The listing builds one solid part. Answer for the finished solid, in the listing's coordinates (mm). Coordinates: 2 decimals unless noted, no trailing zeros. Order: outer loops, then holes, each group sorted by start corner. A loop starts at its lowest first (then second) coordinate and runs counter-clockwise, first axis right, second up.
from build123d import *

# Parameters (mm, degrees)
F0_W     = 8
F0_H     = 8
F0_W_2   = 7.999141
F1_DEPTH = 3
F2_R     = 2.2
F3_DEPTH = 5
F4_R     = 2.5
F5_DEPTH = 6.5


with BuildPart() as f1:
    # F0 (on Top) → F1 (new body)
    with BuildSketch(Plane.XY):
        Polygon((-37.766442, 20.223286), (-40, 20.223286), (-40, -20.223286), (-37.766442, -20.223286), (-29.767301, -20.223286), (29.767301, -20.223286), (37.766442, -20.223286), (40, -20.223286), (40, 20.223286), (37.766442, 20.223286), (36.185599, 20.223286), (29.766442, 20.223286), (28.185599, 20.223286), (-29.766442, 20.223286), align=None)
        with Locations((-33.766442, 24.223286)):
            Rectangle(F0_W, F0_H)
        with Locations((-33.766872, -24.223286)):
            Rectangle(F0_W_2, F0_H)
        Polygon((29.766442, 28.223286), (29.766442, 20.223286), (36.185599, 20.223286), (37.766442, 20.223286), (37.766442, 28.223286), align=None)
        with Locations((33.766872, -24.223286)):
            Rectangle(F0_W_2, F0_H)
    extrude(amount=F1_DEPTH)

    # F2 (on Top) → F3 (cut)
    with BuildSketch(Plane.XY):
        with Locations((-33.882905, 24.085037)):
            Circle(F2_R)
        with Locations((-33.74939, -24.326075)):
            Circle(F2_R)
        with Locations((33.882905, 24.085037)):
            Circle(F2_R)
        with Locations((33.74939, -24.326075)):
            Circle(F2_R)
    extrude(amount=F3_DEPTH, mode=Mode.SUBTRACT)

    # F4 (on Top) → F5 (join)
    with BuildSketch(Plane.XY):
        with Locations((-14.231804, 0)):
            Circle(F4_R)
        with Locations((14.231804, 0)):
            Circle(F4_R)
    extrude(amount=F5_DEPTH)


solid = f1.part
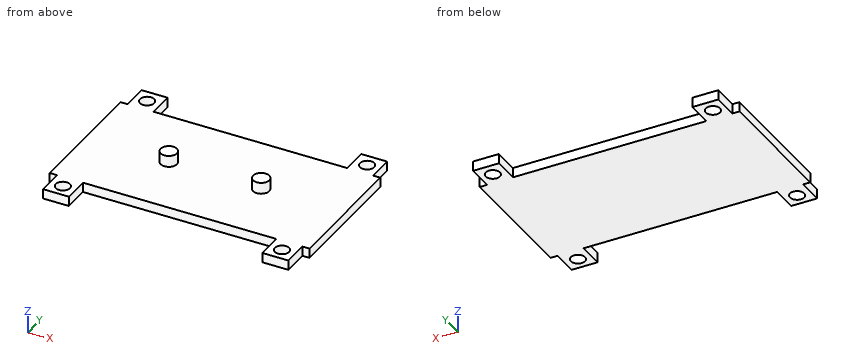
1) Section B-B (z = 1.75) is taken. Give the vertices of the cut face in (x, y).
2) Each of these flat-tipped pins is pushed along its axis until it touches: P1, Ø0.9, axis at y = -24, z = 1.5, coming from the -X side; P2, Ø2, axis at y = 21.5, z = 5, coming from the +X side; P3, Ø0.7, axis at x = 39.5, z = 1, coming from the -Y side; P4, Ø2.5, axis at y = -22.5, z = 1.5, coming from the +X side. Where does it stop, or does it pass through?
3) Consider L1, parallel to X at y = -20.5, z = 2; L2, parallel to Z at x = 21, y = -16; L3, parallel to Y at x = 12.5, z = 1.75. Determine where each line is inside the solid, lowest interval first.
4) Section C-C (x = -25) is taken. Give the vertices of the cut face in (y, z), then the cut area to 3 significant figures.
5) Section A-A (y = 0) is taken. Give the vertices of the cut face in (x, z), then the cut area to 3 significant figures.
6) Section D-D (y = 15) is taken. Give the vertices of the cut face in (x, z).
Filled sheet:
1. outline: (-40, -20.22) - (-37.77, -20.22) - (-37.77, -28.22) - (-29.77, -28.22) - (-29.77, -20.22) - (29.77, -20.22) - (29.77, -28.22) - (37.77, -28.22) - (37.77, -20.22) - (40, -20.22) - (40, 20.22) - (37.77, 20.22) - (37.77, 28.22) - (29.77, 28.22) - (29.77, 20.22) - (-29.77, 20.22) - (-29.77, 28.22) - (-37.77, 28.22) - (-37.77, 20.22) - (-40, 20.22) - close; hole circle Ø4.4 at (-33.88, 24.09); hole circle Ø4.4 at (-33.75, -24.33); hole circle Ø4.4 at (33.75, -24.33); hole circle Ø4.4 at (33.88, 24.09)
2. P1: stops at x = -37.77
2. P2: passes through
2. P3: stops at y = -20.22
2. P4: stops at x = 37.77
3. L1: x = -37.77 to -29.77, 29.77 to 37.77
3. L2: z = 0 to 3
3. L3: y = -20.22 to 20.22
4. outline: (-20.22, 0) - (20.22, 0) - (20.22, 3) - (-20.22, 3) - close
4. area: 121 mm2
5. outline: (-40, 0) - (40, 0) - (40, 3) - (16.73, 3) - (16.73, 6.5) - (11.73, 6.5) - (11.73, 3) - (-11.73, 3) - (-11.73, 6.5) - (-16.73, 6.5) - (-16.73, 3) - (-40, 3) - close
5. area: 275 mm2
6. outline: (-40, 0) - (40, 0) - (40, 3) - (-40, 3) - close
